Model file for the job. Use its own axes, mm. Face numbers are marked on the shaded views. A direction names the side the tool comes from. Give positions to 0.01 mm unless a question says otherwise; leave off trailing zeros. Loops run counter-clockwise (first coordinate to the right, second up) from the corner with the lowest first, then second, coordinate; pieces in that order, holes last. Notation, with made-up numbers: (70.25, 65.25) - (85.25, 65.25) arc R14 ccw to (85.25, 70.25) - close; hole circle Ø2 at (5, -7.75). An arc over 180 degrees is marked (long way). Use a Markdown table: item, result.
from build123d import *

# Parameters (mm, degrees)
SKETCH2_W           = 12.4
SKETCH2_H           = 10
SKETCH2_W_2         = 7.6
BOSS_EXTRUDE1_DEPTH = 5
SKETCH3_R           = 0.925
CUT_EXTRUDE1_DEPTH  = 10
SKETCH4_W           = 4
SKETCH4_H           = 10
BOSS_EXTRUDE2_DEPTH = 10
FILLET1_R           = 2
SKETCH5_R           = 1
CUT_EXTRUDE2_DEPTH  = 4


with BuildPart() as part:
    # Sketch2 → Boss-Extrude1 (new body)
    with BuildSketch(Plane(origin=(-29.355490461, 0, 0), x_dir=(0, 0, -1), z_dir=(1, 0, 0))):
        with Locations((6.2, -11)):
            Rectangle(SKETCH2_W, SKETCH2_H)
        with Locations((16.2, -11)):
            Rectangle(SKETCH2_W_2, SKETCH2_H)
    extrude(amount=BOSS_EXTRUDE1_DEPTH)

    # Sketch3 → Cut-Extrude1 (cut)
    with BuildSketch(Plane(origin=(0, -16, 0), x_dir=(-1, 0, 0), z_dir=(0, -1, 0))):
        with Locations(Location((26.755490461, 6.2, 0), (0, 0, 90))):
            Circle(SKETCH3_R)
    extrude(amount=-CUT_EXTRUDE1_DEPTH, mode=Mode.SUBTRACT)

    # Sketch4 → Boss-Extrude2 (add)
    with BuildSketch(Plane(origin=(-24.355490461, 0, 0), x_dir=(0, 0, -1), z_dir=(1, 0, 0))):
        with Locations((18, -11)):
            Rectangle(SKETCH4_W, SKETCH4_H)
    extrude(amount=BOSS_EXTRUDE2_DEPTH)

    # Fillet1
    fillet1_edges = [part.edges().sort_by_distance(p)[0] for p in [
        (-24.355490461, -11, 0),
        (-24.355490461, -11, -16),
        (-14.355490461, -11, -16),
    ]]
    fillet(fillet1_edges, radius=FILLET1_R)

    # Sketch5 → Cut-Extrude2 (cut)
    with BuildSketch(Plane.XY.offset(-16)):
        with Locations((-19.355490461, -8.5)):
            Circle(SKETCH5_R)
        with Locations((-19.355490461, -13.5)):
            Circle(SKETCH5_R)
    extrude(amount=-CUT_EXTRUDE2_DEPTH, mode=Mode.SUBTRACT)


solid = part.part
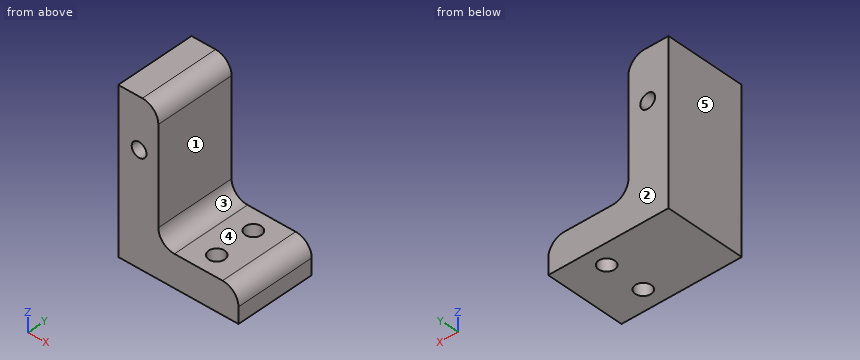
(1) Slice it at A-A, the plane z = -6.2. Write the cut outline in (x, y), plus the area to 3 significant figures.
Computed:
| item | result |
|---|---|
| outline | (-29.36, -16) - (-27.68, -16) - (-27.68, -6) - (-29.36, -6) - close; (-25.83, -16) - (-24.36, -16) - (-24.36, -6) - (-25.83, -6) - close |
| area | 31.5 mm² |
(2) Mould opens along X. For the marked faces 3, 4 and 5 say: pulls with the +X half, pulls with the -X half, needs draft (parallel to the pull), parting line crosses it, or undercut.
Computed:
| item | result |
|---|---|
| face 3 | pulls with the +X half |
| face 4 | needs draft |
| face 5 | pulls with the -X half |
(3) Slice it at C-C, the plane x = -27. Write the cut outline in (y, z), plus the area to 3 significant figures.
Computed:
| item | result |
|---|---|
| outline | (-16, -20) - (-6, -20) - (-6, -7.09) - (-16, -7.09) - close; (-16, -5.31) - (-6, -5.31) - (-6, 0) - (-16, 0) - close |
| area | 182 mm² |
(4) 3-axis set-ups, long thin cutter, end or side, ignore diameter. For the marked faces 1 and 2: which of +Z, -Z, +X, -X, +Y, -Y reach the whole face in a straight line?
Computed:
| item | result |
|---|---|
| face 1 | +Z, +X, +Y, -Y |
| face 2 | +Z, -Z, +X, -X, +Y |
(5) Pin check, flat tips, straight feed: P1, Ø6, axis at x = -21, y = -12, coming from the +Z side; P2, Ø3, axis at x = -18.5, y = -10.5, coming from the +Z side; P3, Ø3, axis at y = -8.5, z = -8.5, coming from the +X side. Stop position of each tip, or through.
Computed:
| item | result |
|---|---|
| P1 | z = -15.14 |
| P2 | z = -16 |
| P3 | x = -24.36 |
(6) Slice it at B-B, the plane y = -13.5. Count the separate pieces of the cut face and the enclosed holes in it, plus the area to 3 significant figures.
Computed:
| item | result |
|---|---|
| separate pieces | 2 |
| enclosed holes | 1 |
| area | 128 mm² |
(7) Drill centre lines: probe 1 along X at (y, z) = (-13, -6.2); probe 2 along X at (y, z) = (-10, -3.75); probe 3 along Z at (x, y) = (-17, -15). Where is each one in solid material? Low to high. Write a range as [from, to].
Computed:
| item | result |
|---|---|
| probe 1 | [-29.36, -27.68], [-25.83, -24.36] |
| probe 2 | [-29.36, -24.36] |
| probe 3 | [-20, -16] |
